Geometry: see drawing. Coordinates: mm, zero at the bounding-box minimum. A direction names the side the tool comes from. Give positions to 0.01 mm unless a question says otherwise; leave off trailing zeros. Write each loop counter-clockwise with the first axis right and the second up, starting at its lowest first coordinate (ties: lowest second). Pieces come first, ordered by that corner, then holes. Notation, with made-up numbers: (16.5, 55) -> (48.5, 55) arc R27 cw to (48.5, 79) -> close; hole circle Ø7 at (-1.5, -31). An arc over 180 degrees is marked (long way). Use one line per item in the form item = value. Start each with the question number.
(1) Cut plane D-D, the plane y = 7.25. Output: boundary loops of the cut face in (x, z).
(2) Material intervals for line 1 along X through (y, z) = (8, 2.85); line 2 along X through (y, z) = (1.75, 2.2); line 3 along Y through (x, z) = (10.25, 1.8), sorted ascending. Write a range as from..to.
(3) Set-up query: the marked faces 4, 5 and 6. Return all of +Z, -Z, +X, -X, +Y, -Y with unobstructed straight access to the full face (end or side cutting, diameter ignored); none if empty.
(4) Draft query along Y for the marked faces 1, 2 and 3. Return one class per face: pulls with the +Y half, pulls with the -Y half, needs draft (parallel to the pull), parting line crosses it, or undercut.
(5) Cut plane B-B, the plane y = 14. Output: boundary loops of the cut face in (x, z).
(6) Cut plane A-A, the plane z = 2.2. Output: boundary loops of the cut face in (x, y), and give its area (3 significant figures).
(7) First-contact query: P1, Ø0.9, axis at y = 7, z = 2, coming from the +X side; P2, Ø1.5, axis at y = 1.5, z = 1.5, coming from the -X side; P3, Ø1.2, axis at x = 6.5, z = 2, coming from the -Y side. Flat tips, straight axial feed; report the tip coordinate or a pass-through.
(8) Cut plane C-C, the plane x = 7.25. Output: boundary loops of the cut face in (y, z).
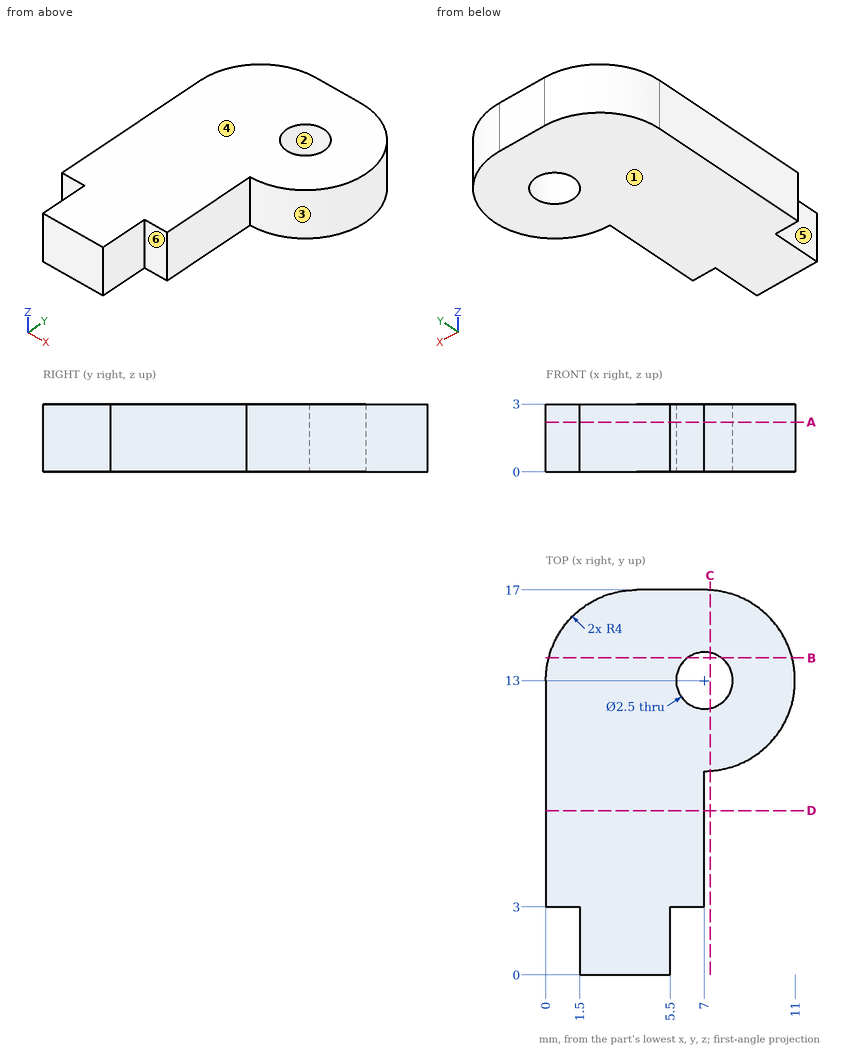
Geometry says:
q1.outline = (0, 0) -> (7, 0) -> (7, 3) -> (0, 3) -> close
q2.line_1 = 0..7
q2.line_2 = 1.5..5.5
q2.line_3 = 10.67..15.33
q3.face_4 = +Z, +X, -X, +Y, -Y
q3.face_5 = +Z, -Z, -X, -Y
q3.face_6 = +Z, -Z, +X, -Y
q4.face_1 = needs draft
q4.face_2 = undercut
q4.face_3 = parting line crosses it
q5.outline = (0.13, 0) -> (6.25, 0) -> (6.25, 3) -> (0.13, 3) -> close; (7.75, 0) -> (10.87, 0) -> (10.87, 3) -> (7.75, 3) -> close
q6.outline = (0, 3) -> (1.5, 3) -> (1.5, 0) -> (5.5, 0) -> (5.5, 3) -> (7, 3) -> (7, 9) arc R4 ccw to (7, 17) -> (4, 17) arc R4 ccw to (0, 13) -> close; hole circle Ø2.5 at (7, 13)
q6.area = 127 mm^2
q7.P1 = 7
q7.P2 = 1.5
q7.P3 = 3
q8.outline = (9.01, 0) -> (11.78, 0) -> (11.78, 3) -> (9.01, 3) -> close; (14.22, 0) -> (16.99, 0) -> (16.99, 3) -> (14.22, 3) -> close
